Autodesk Inventor part; units mm, degrees
ref_plane "YZ Plane" through (0, 0, 0) normal (1, 0, 0) x (0, 1, 0)
ref_plane "XZ Plane" through (0, 0, 0) normal (0, 1, 0) x (-1, 0, 0)
ref_plane "XY Plane" through (0, 0, 0) normal (0, 0, 1) x (1, 0, 0)
sketch "Sketch1" plane through (0, 0, 0) normal (0, 0, 1) x (1, 0, 0)
  line L0 (0, 4.2) -> (0, -4.2)
  line L1 (-4.2, 0) -> (4.2, 0)
  circle A0 centre (0, 0) radius 3
  dimension "d0" = 6
extrude "Extrusion1" add sketch "Sketch1" along normal mid plane 40
chamfer "Chamfer1" distance 1 angle 30 1 edges at (-3, 0, -20) measured on face at (-0.5351, 1.0949, -20)
fillet "Fillet1" radius 0.5 1 edges at (-3, 0, 20)
sketch "Sketch2" plane through (0, 0, 20) normal (0, 0, 1) x (1, 0, 0)
  circle A0 centre (0, 0) radius 2.5
hole "Hole1" at (0, 0, 20) direction (0, 0, -1) diameter 3.242 depth 8 tip angle 118
chamfer "Chamfer2" distance 0.25 angle 45 1 edges at (0, 1.621, 20)
properties part number "PIN, DOWEL, PULL, 6MMODX40MM" material "Steel, 4140, Carb & Case Harden 58-60 Rc, 0.06 Dp Case"
Verification items for the finished model (mm, model axes). A direction names the side the tool comes from. Give positions to 0.01 mm unless a question says otherwise; leave off trailing zeros. Order: outer loops, then holes, each group sorted by start corner. A loop starts at its lowest first (then second) coordinate and runs counter-clockwise, first axis right, second up. Notation, with made-up numbers: M -1,13.25 L 28,13.25 A21 cw 28,24.25 Z; hole C 3.25,22.25 d3. An arc over 180 degrees is marked long. Return JSON: item names as keys, results as strings. Group by question number.
1) Go/stop test with flat-tipped pins: pin 1 Ø1 at (x, z) = (1, 4.5) entering from +Y; pin 2 Ø3 at (x, y) = (0, 0) entering from +Z; pin 3 Ø1.5 at (y, z) = (-2, -14.5) entering from -X. Record where each tip stops, or that it passes through.
2) Section check A-A on z = -16.5. Record the cut outline in (x, y).
3) Scan lines: line 1 (Y direction, x = 0, z = 17.75); line 2 (Z direction, x = -1.8, y = 0.5). Record each from-to range of solid material in increasing order.
4) Mould release check, pull along X, two halves, no side actions. Record for faces 3 (the face through (1, -2, 20)), 4 (the face through (-0.275, 0.061, 11.195)), 5 (the face through (-3, 0, 0)): pulls with the +X half, pulls with the -X half, needs draft (parallel to the pull), parting line crosses it, or undercut.
5) Access from +Z, -Z, +X, -X, +Y, -Y to the whole of each face (thin tool, end or side, straight path). Record for faces 1 (the face through (1.438, -0.748, 15.821)), 2 (the face through (0, 0, -20)).
Answer block:
{
 "1": {"pin 1": "stops at y = 2.96", "pin 2": "stops at z = 11.93", "pin 3": "stops at x = -2.73"},
 "2": {"outline": "C 0,0 d6"},
 "3": {"line 1": "y = -3 to -1.62, 1.62 to 3", "line 2": "z = -20 to 20"},
 "4": {"face 3": "needs draft", "face 4": "undercut", "face 5": "parting line crosses it"},
 "5": {"face 1": "+Z", "face 2": "-Z, +X, -X, +Y, -Y"}
}
